Build history of the part. All positions in model axes, mm. A direction names the side the tool comes from. Give positions to 0.01 mm unless a question says otherwise; leave off trailing zeros. Loops run counter-clockwise (first coordinate to the right, second up) from the corner with the lowest first, then second, coordinate; pieces in that order, holes last. Notation, with made-up numbers: M -6,-20.5 L 50,-20.5 A21 ccw 50,13.5 Z; hole C 43,7.25 d6. An arc over 180 degrees is marked long. Answer in a Markdown table with one row per item. Add a question column.
```python
from build123d import *

# Parameters (mm, degrees)
SKETCH_1_R         = 1.25
BOARD_DEPTH        = 1
SKETCH_2_W         = 38
SKETCH_2_H         = 30
SCREEN_DEPTH       = 2
SCREEN_RADIUS_R    = 3.5
SCREEN_TOP_START   = 0.1
SCREEN_TOP_DEPTH   = 0.1
SKETCH_3_W         = 51
SKETCH_3_H         = 5
PLUG_DEPTH         = 5.2
SKETCH_4_W         = 15.14
SKETCH_4_H         = 20
SPEAKER_DEPTH      = 5
SKETCH_10_W        = 8
SKETCH_10_H        = 6
SPEAKER2PLUG_DEPTH = 5.5
SKETCH_5_W         = 12.7
SKETCH_5_H         = 6
BUTTON_DEPTH       = 6
SKETCH_6_W         = 1
SKETCH_6_H         = 4
BUTTON_TAP_DEPTH   = 1
TAP_RADIUS_R       = 0.6
SKETCH_7_W         = 1.5
SKETCH_7_H         = 1.5
RGB_LED_DEPTH      = 0.7
SKETCH_8_W         = 3.2
SKETCH_8_H         = 2.5
MIC_DEPTH          = 1.3
SKETCH_11_W        = 26.2
SKETCH_11_H        = 0.1
SPLIT_2_DEPTH      = 1


with BuildPart() as part:
    # 草图1 → board (new body)
    with BuildSketch(Plane(origin=(0, 0, 0), x_dir=(1, 0, 0), z_dir=(0, 1, 0))):
        with BuildLine():
            Line((-29, 15), (29, 15))
            ThreePointArc((29, 15), (31.474873734, 13.974873734), (32.5, 11.5))
            Line((32.5, 11.5), (32.5, -11.5))
            ThreePointArc((32.5, -11.5), (31.474873734, -13.974873734), (29, -15))
            Line((29, -15), (-29, -15))
            ThreePointArc((-29, -15), (-31.474873734, -13.974873734), (-32.5, -11.5))
            Line((-32.5, -11.5), (-32.5, 11.5))
            ThreePointArc((-32.5, 11.5), (-31.474873734, 13.974873734), (-29, 15))
        make_face()
        with Locations(Location((-29, 11.5, 0), (0, 0, 270))):
            Circle(SKETCH_1_R, mode=Mode.SUBTRACT)
        with Locations(Location((29, 11.5, 0), (0, 0, 270))):
            Circle(SKETCH_1_R, mode=Mode.SUBTRACT)
        with Locations(Location((-29, -11.5, 0), (0, 0, 270))):
            Circle(SKETCH_1_R, mode=Mode.SUBTRACT)
        with Locations(Location((29, -11.5, 0), (0, 0, 270))):
            Circle(SKETCH_1_R, mode=Mode.SUBTRACT)
    extrude(amount=BOARD_DEPTH)

    # 草图2 → screen (add)
    with BuildSketch(Plane(origin=(0, 1, 0), x_dir=(1, 0, 0), z_dir=(0, 1, 0))):
        with Locations((7.5, 0)):
            Rectangle(SKETCH_2_W, SKETCH_2_H)
    extrude(amount=SCREEN_DEPTH)

    # screen-radius
    screen_radius_edges = [part.edges().sort_by_distance(p)[0] for p in [
        (-11.5, 2, -15),
        (-11.5, 2, 15),
        (26.5, 2, 15),
        (26.5, 2, -15),
    ]]
    fillet(screen_radius_edges, radius=SCREEN_RADIUS_R)

    # 草图9 → screen-top (add)
    with BuildSketch(Plane(origin=(0, 3, 0), x_dir=(1, 0, 0), z_dir=(0, 1, 0)).offset(SCREEN_TOP_START)):
        with BuildLine():
            Line((26.5, -11.5), (26.5, 11.5))
            ThreePointArc((26.5, 11.5), (25.80624304, 13.591650066), (24, 14.854101966))
            Line((24, 14.854101966), (24, -14.854101966))
            ThreePointArc((24, -14.854101966), (25.80624304, -13.591650066), (26.5, -11.5))
        make_face()
    extrude(amount=-SCREEN_TOP_DEPTH)

    # 草图3 → plug (add)
    with BuildSketch(Plane.XZ):
        with Locations((0, -11.75)):
            Rectangle(SKETCH_3_W, SKETCH_3_H)
    extrude(amount=PLUG_DEPTH)

    # 草图4 → speaker (add)
    with BuildSketch(Plane.XZ):
        with Locations((-17.52, 2.68)):
            Rectangle(SKETCH_4_W, SKETCH_4_H)
    extrude(amount=SPEAKER_DEPTH)

    # 草图10 → speaker2plug (add)
    with BuildSketch(Plane.XZ):
        with Locations((-4, 12)):
            Rectangle(SKETCH_10_W, SKETCH_10_H)
    extrude(amount=SPEAKER2PLUG_DEPTH)

    # 草图5 → button (add)
    with BuildSketch(Plane.XZ):
        with Locations((11.85, 12)):
            Rectangle(SKETCH_5_W, SKETCH_5_H)
    extrude(amount=BUTTON_DEPTH)

    # 草图6 → button-tap (add)
    with BuildSketch(Plane.XY.offset(15)):
        with Locations((9.5, -3)):
            Rectangle(SKETCH_6_W, SKETCH_6_H)
    extrude(amount=BUTTON_TAP_DEPTH)

    # tap-radius
    # the kernel refuses this fillet: 0.6 mm, written as the material it takes off along each edge
    with BuildSketch(Plane(origin=(10, 0.5, 16), x_dir=(0, 0, -1), z_dir=(0, -1, 0)), Plane(origin=(9, -6.5, 16), x_dir=(0, 0, -1), z_dir=(0, 1, 0))) as tap_radius_piece_1:
        with BuildLine():
            CenterArc((TAP_RADIUS_R, -TAP_RADIUS_R), TAP_RADIUS_R, 90, 90)
            Line((0, -TAP_RADIUS_R), (0, 0))
            Line((0, 0), (TAP_RADIUS_R, 0))
        make_face()
    extrude(amount=7, mode=Mode.SUBTRACT)

    # 草图7 → rgb-led (add)
    with BuildSketch(Plane(origin=(0, 1, 0), x_dir=(1, 0, 0), z_dir=(0, 1, 0))):
        with Locations((29.25, 0)):
            Rectangle(SKETCH_7_W, SKETCH_7_H)
    extrude(amount=RGB_LED_DEPTH)

    # 草图8 → mic (add)
    with BuildSketch(Plane(origin=(0, 1, 0), x_dir=(1, 0, 0), z_dir=(0, 1, 0))):
        with Locations((-26.6, -0.25)):
            Rectangle(SKETCH_8_W, SKETCH_8_H)
    extrude(amount=MIC_DEPTH)

    # 草图11 → split 2 (cut)
    with BuildSketch(Plane.XY.offset(15)):
        with Locations((5.1, -0.05)):
            Rectangle(SKETCH_11_W, SKETCH_11_H)
    extrude(amount=-SPLIT_2_DEPTH, mode=Mode.SUBTRACT)


solid = part.part
```
(1) Slice it at A-A, the plane y = -3.5. Give the cut face in (x, z).
(2) Slice it at D-D, the plane z = 0. Give the cut face in (x, y).
(3) Slice it at B-B, the plane z = 5.5. Give the cut face in (x, y), then the cut area to 3 significant figures.
(4) Pin check, flat tips, straight feed: pin 1 (6 mm diameter, centred on x = -8.5, z = 5, fed in from +Y); pin 2 (4 mm diameter, centred on x = -9, y = -1, fed in from +Z); pin 3 (4 mm diameter, centred on x = -18.5, z = 2, fed in from -Y); pin 4 (2.5 mm diameter, centred on y = 2, z = -1.5, fed in from +X). Stop position of each tip, or through.
(5) Tool access for faces 5 (the flat face through (-27, 2, 1.5)), 6 (the flat face through (-18, -2, 12.68)), 7 (the flat face through (-27, 2, -1)), 8 (the flat face through (18.2, -3, 12)), 9 (the flat face through (0, -3, -14.25)): list every direction of +Z, -Z, +X, -X, +Y, -Y with a clear straight run to the whole face (end or side of a thin tool).
(6) Pull direction X, two halves, no side cores. Call faces 1 (the flat face through (-28.2, 2, 0)), 2 (the cylindrical face through (29.05, 0.49, -12.75)), 3 (the flat face through (-8, -3, 12)), 4 (the flat face through (-27, 2.3, 0)): +X half, -X half, draft (parallel to the pull), parting line (faces both ways), or undercut.
(7) Wall check: line 1 (X direction, y = -2.5, z = 11); line 2 (X direction, y = 0.65, z = -11.5); line 3 (Z direction, x = -17.5, y = -4.75). Give the ranges that are in metal, low to high.
(8) Slice it at C-C, the plane x = -3.5. Give the cut face in (y, z), then the cut area to 3 significant figures.
Solution:
| question | item | result |
|---|---|---|
| 1 | outline | M -25.5,-14.25 L 25.5,-14.25 L 25.5,-9.25 L -25.5,-9.25 Z; M -25.09,-7.32 L -9.95,-7.32 L -9.95,12.68 L -25.09,12.68 Z; M -8,9 L 0,9 L 0,15 L -8,15 Z; M 5.5,9 L 18.2,9 L 18.2,15 L 10,15 L 10,15.4 A0.6 ccw 9.5,15.99 A0.6 ccw 9,15.4 L 9,15 L 5.5,15 Z |
| 2 | outline | M -32.5,0 L -25.09,0 L -25.09,-5 L -9.95,-5 L -9.95,0 L 32.5,0 L 32.5,1 L 30,1 L 30,1.7 L 28.5,1.7 L 28.5,1 L 26.5,1 L 26.5,3.1 L 24,3.1 L 24,3 L -11.5,3 L -11.5,1 L -25,1 L -25,2.3 L -28.2,2.3 L -28.2,1 L -32.5,1 Z |
| 3 | outline | M -32.5,0 L -25.09,0 L -25.09,-5 L -9.95,-5 L -9.95,0 L 32.5,0 L 32.5,1 L 26.5,1 L 26.5,3.1 L 24,3.1 L 24,3 L -11.5,3 L -11.5,1 L -32.5,1 Z |
| 3 | area | 217 mm^2 |
| 4 | pin 1 | y = 3 |
| 4 | pin 2 | z = 15 |
| 4 | pin 3 | y = -5 |
| 4 | pin 4 | x = 32.5 |
| 5 | face 5 | +Z, -X, +Y |
| 5 | face 6 | +Z, -X, -Y |
| 5 | face 7 | -Z, -X, +Y |
| 5 | face 8 | +Z, +X, -Y |
| 5 | face 9 | -Z, +X, -X, -Y |
| 6 | face 1 | -X half |
| 6 | face 2 | undercut |
| 6 | face 3 | undercut |
| 6 | face 4 | draft |
| 7 | line 1 | -25.09 to -9.95, -8 to 0, 5.5 to 18.2 |
| 7 | line 2 | -32.5 to -30.25, -27.75 to 27.75, 30.25 to 32.5 |
| 7 | line 3 | -14.25 to -9.25, -7.32 to 12.68 |
| 8 | outline | M -5.5,9 L 0,9 L 0,-9.25 L -5.2,-9.25 L -5.2,-14.25 L 0,-14.25 L 0,-15 L 3,-15 L 3,15 L 0,15 L 0,14 L -0.1,14 L -0.1,15 L -5.5,15 Z |
| 8 | area | 149 mm^2 |
